Check sheet for the drawn part. Datum: minimum x, y, z corner. Units: mm. A direction names the side the tool comes from. Coordinates: 2 decimals unless noted, no trailing zeros. Order: outer loops, then holes, each group sorted by start corner. A loop starts at its lowest first (then second) coordinate and runs counter-clockwise, first axis right, second up. Notation, with made-up numbers: M 69,-38.5 L 82,-38.5 A24 ccw 82,-19.5 Z; hole C 39,46 d6. An arc over 180 degrees is marked long. Answer in a Markdown table with one row per item. Add a question column.
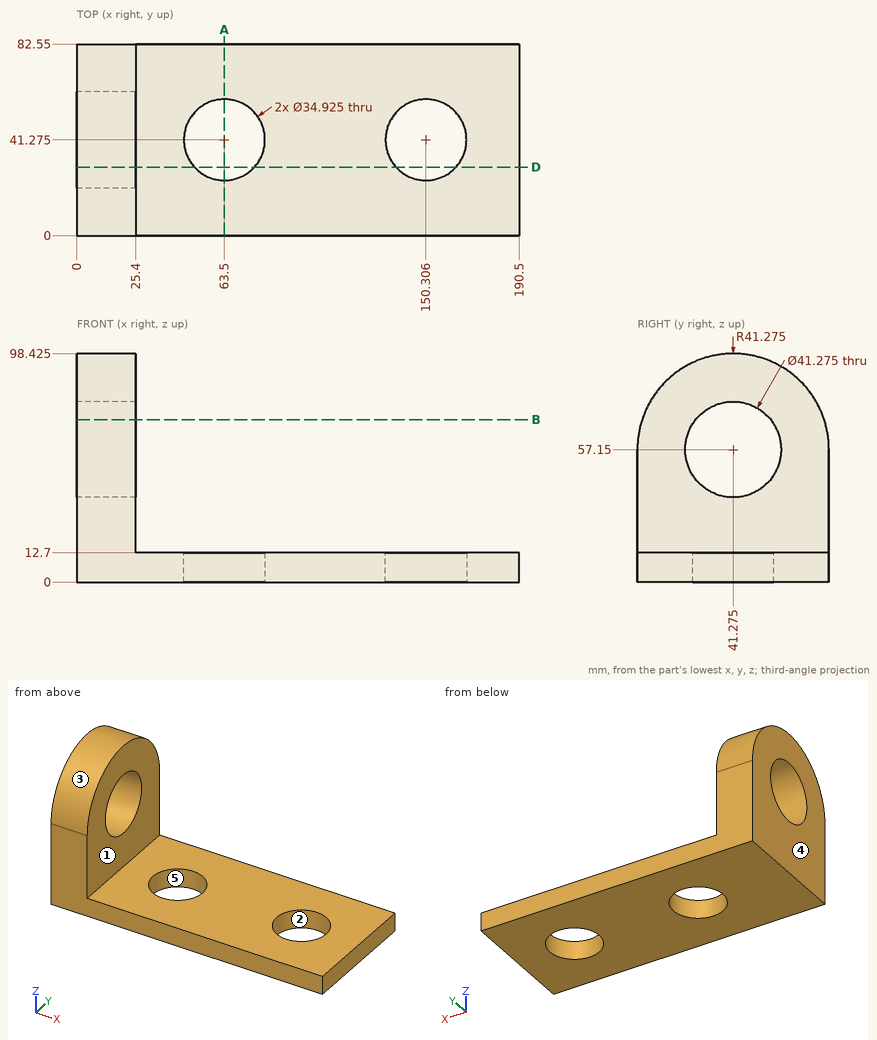
1. Go/stop test with flat-tipped pins: pin 1 Ø25 at (y, z) = (30.5, 70.5) entering from +X; pin 2 Ø6 at (x, y) = (164, 48.5) entering from +Z. Record where each tip stops, or that it passes through.
2. Section check B-B on z = 70. Enter the section's corners in (x, y), then the cut area to 3 significant figures.
3. Section check A-A on x = 63.5. Enter the section's corners in (y, z), then the cut area to 3 significant figures.
4. Set-up check for the marked faces 1 and 2: record each of +Z, -Z, +X, -X, +Y, -Y from which the full face is reachable in a straight line by a thin tool's end or side.
5. Section check D-D on y = 29.5. Enter the section's corners in (x, z) (1 decimal).
6. Scan lines: line 1 (Y direction, x = 14, z = 57); line 2 (Y direction, x = 63.5, z = 6.75); line 3 (Z direction, x = 118.5, y = 62). Record each from-to range of solid material in increasing order.
7. Release check for a two-part mould opening along X. For the marked faces 3, 4 and 5 record: released by +X, released by -X, zero draft, split by the parting line, or undercut.
Result sheet:
| question | item | result |
|---|---|---|
| 1 | pin 1 | x = 25.4 |
| 1 | pin 2 | z = 12.7 |
| 2 | outline | M 0,2.05 L 25.4,2.05 L 25.4,25.13 L 0,25.13 Z; M 0,57.42 L 25.4,57.42 L 25.4,80.5 L 0,80.5 Z |
| 2 | area | 1,170 mm^2 |
| 3 | outline | M 0,0 L 23.81,0 L 23.81,12.7 L 0,12.7 Z; M 58.74,0 L 82.55,0 L 82.55,12.7 L 58.74,12.7 Z |
| 3 | area | 605 mm^2 |
| 4 | face 1 | +Z, +X, +Y, -Y |
| 4 | face 2 | +Z, -Z |
| 5 | outline | M 0,0 L 50.6,0 L 50.6,12.7 L 25.4,12.7 L 25.4,40.2 L 0,40.2 Z; M 0,74.1 L 25.4,74.1 L 25.4,96.7 L 0,96.7 Z; M 76.4,0 L 137.4,0 L 137.4,12.7 L 76.4,12.7 Z; M 163.2,0 L 190.5,0 L 190.5,12.7 L 163.2,12.7 Z |
| 6 | line 1 | 0 to 20.64, 61.91 to 82.55 |
| 6 | line 2 | 0 to 23.81, 58.74 to 82.55 |
| 6 | line 3 | 0 to 12.7 |
| 7 | face 3 | zero draft |
| 7 | face 4 | released by -X |
| 7 | face 5 | undercut |
